The listing builds one solid part. Answer for the finished solid, in the listing's coordinates (mm). Round coordinates to 2 decimals unless told otherwise and drop trailing zeros. Order: outer loops, then holes, each group sorted by start corner. A loop starts at its lowest first (then second) coordinate and runs counter-clockwise, first axis right, second up. Notation, with made-up numbers: (6.25, 37) - (51.25, 37) arc R21 cw to (51.25, 53) - close; hole circle Ø8 at (5.5, 40). An arc over 180 degrees is marked (long way). Write item = value, one per line.
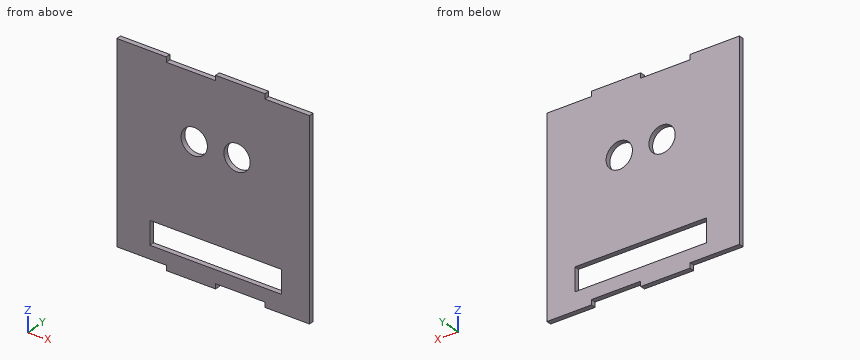
from build123d import *

# Parameters (mm, degrees)
F0_W     = 80
F0_H     = 14
F0_R     = 8
F1_DEPTH = 1.5


# Not quite as in the source:
# - a feature names something its author has since deleted; it is built from what else it names


with BuildPart() as f1:
    # F0 (on Front) → F1 (new body, symmetric)
    with BuildSketch(Plane.XZ):
        Polygon((-30, -2.9994321861), (0, -2.9994321861), (0, 0), (30, 0), (30, -2.9994321861), (57, -2.9994321861), (57, 114.0005678139), (30, 114.0005678139), (30, 117.0005678139), (0, 117.0005678139), (0, 114.0005678139), (-30, 114.0005678139), (-30, 117.0005678139), (-60, 117.0005678139), (-60, 0), (-30, 0), align=None)
        with Locations((0, 14.8116284981)):
            Rectangle(F0_W, F0_H, mode=Mode.SUBTRACT)
        with Locations((-13, 75.2281695604)):
            Circle(F0_R, mode=Mode.SUBTRACT)
        with Locations((13, 75.2218647463)):
            Circle(F0_R, mode=Mode.SUBTRACT)
    extrude(amount=F1_DEPTH, both=True)


solid = f1.part
Q1. Section A-A on x = -13 is taken. Determine the outline of the cut face in (y, z), then the cut area to 3 significant figures.
Model answer:
outline = (-1.5, -3) - (1.5, -3) - (1.5, 7.81) - (-1.5, 7.81) - close; (-1.5, 21.81) - (1.5, 21.81) - (1.5, 67.23) - (-1.5, 67.23) - close; (-1.5, 83.23) - (1.5, 83.23) - (1.5, 114) - (-1.5, 114) - close
area = 261 mm^2
Q2. Section D-D on x = 13 is taken. Determine the outline of the cut face in (y, z), then the cut area to 3 significant figures.
Model answer:
outline = (-1.5, 0) - (1.5, 0) - (1.5, 7.81) - (-1.5, 7.81) - close; (-1.5, 21.81) - (1.5, 21.81) - (1.5, 67.22) - (-1.5, 67.22) - close; (-1.5, 83.22) - (1.5, 83.22) - (1.5, 117) - (-1.5, 117) - close
area = 261 mm^2
Q3. Section C-C on y = -0.45 is taken. Determine the outline of the cut face in (x, z), then the cut area to 3 significant figures.
Model answer:
outline = (-60, 0) - (-30, 0) - (-30, -3) - (0, -3) - (0, 0) - (30, 0) - (30, -3) - (57, -3) - (57, 114) - (30, 114) - (30, 117) - (0, 117) - (0, 114) - (-30, 114) - (-30, 117) - (-60, 117) - close; hole (-40, 7.81) - (40, 7.81) - (40, 21.81) - (-40, 21.81) - close; hole circle Ø16 at (-13, 75.23); hole circle Ø16 at (13, 75.22)
area = 12,200 mm^2
Q4. Section B-B on x = 32.5 is taken. Determine the outline of the cut face in (y, z).
Model answer:
outline = (-1.5, -3) - (1.5, -3) - (1.5, 7.81) - (-1.5, 7.81) - close; (-1.5, 21.81) - (1.5, 21.81) - (1.5, 114) - (-1.5, 114) - close
Q5. Find the intervals of material crossed by line 1 (Z direction, x = 13, y = 0.3); line 2 (Z direction, x = -12.5, y = 0.4); line 3 (Z direction, x = 2, y = 0.2), in increasing order. Write a range as from..to.
Model answer:
line_1 = 0..7.81, 21.81..67.22, 83.22..117
line_2 = -3..7.81, 21.81..67.24, 83.21..114
line_3 = 0..7.81, 21.81..117
Q6. Flat-ended cylindrical pins translate along their axes: P1, Ø13, axis at x = -13, z = 75.23, coming from the +Y side; P2, Ø0.9, axis at x = 17.5, y = 0.5, coming from the -Z side; P3, Ø1.5, axis at y = 0.5, z = -2, coming from the -X side. Find the tip coordinate at first contact, or state that the pin passes through.
Model answer:
P1 = through
P2 = 0
P3 = -30
